Input: part model. Units: mm. Frame: model coordinates. Coordinates: 2 decimals unless noted, no trailing zeros. Loops run counter-clockwise (first coordinate to the right, second up) from the corner with the lowest first, then second, coordinate; pieces in that order, holes last. Notation, with made-up numbers: (-36, -6) - (-22, -6) arc R8 ccw to (-22, 8) - close; hole circle Ø3 at (-6, 43.25). An arc over 180 degrees is marked (long way). Answer as CSV lines item,"result". Start each with the question number.
Autodesk Inventor part; units mm, degrees
ref_plane "YZ Plane" through (0, 0, 0) normal (1, 0, 0) x (0, 1, 0)
ref_plane "XZ Plane" through (0, 0, 0) normal (0, 1, 0) x (-1, 0, 0)
ref_plane "XY Plane" through (0, 0, 0) normal (0, 0, 1) x (1, 0, 0)
sketch "Sketch2" plane through (0, 0, 0) normal (0, 1, 0) x (-1, 0, 0)
  line L0 (0, 0) -> (300, 0)
  line L1 (300, 0) -> (300, -500)
  line L2 (300, -500) -> (0, -500)
  line L3 (0, -500) -> (0, 0)
  line L4 (300, 0) -> (255, 0)
  line L5 (255, 0) -> (255, -45)
  line L6 (255, -45) -> (300, -45)
  line L7 (300, -45) -> (300, 0)
  line L8 (300, -500) -> (255, -500)
  line L9 (255, -500) -> (255, -455)
  line L10 (255, -455) -> (300, -455)
  line L11 (300, -455) -> (300, -500)
  line L12 (0, -500) -> (45, -500)
  line L13 (45, -500) -> (45, -455)
  line L14 (45, -455) -> (0, -455)
  line L15 (0, -455) -> (0, -500)
  line L16 (0, 0) -> (45, 0)
  line L17 (45, 0) -> (45, -45)
  line L18 (45, -45) -> (0, -45)
  line L19 (0, -45) -> (0, 0)
  point P0 (0, -45)
  point P1 (0, -455)
  point P2 (300, -455)
  point P3 (255, 0)
  point P4 (45, 0)
  dimension "d0" = 300
  dimension "d1" = 500
  dimension "d12" = 45
  dimension "d13" = 45
  dimension "d14" = 45
  dimension "d15" = 45
  dimension "d16" = 45
  dimension "d17" = 45
  dimension "d18" = 45
  dimension "d19" = 45
ref_plane "Work Plane1" through (0, 20, 0) normal (0, 1, 0) x (1, 0, 0)
extrude "Extrusion2" add sketch "Sketch2" along normal blind 20 contours L0 L5 L6 L1 L10 L9 L2 L13 L14 L3 L18 L17
properties part number "Shelf"
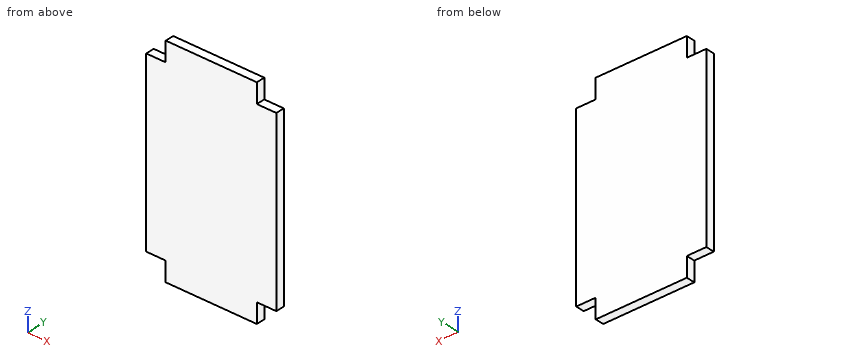
Item 1: Section query A-A, the plane y = 3.5. Output: boundary loops of the cut face in (x, z), and give its area (3 significant figures).
Item 2: Material intervals for probe 1 along X at (y, z) = (11.5, -36.5); probe 2 along Z at (x, y) = (-42, 13.5), sorted ascending.
Item 3: Section query B-B, the plane x = -266.5. Output: boundary loops of the cut face in (y, z).
Item 4: Contact query for flat-ended pins moving along their axis: P1, Ø12, axis at x = -269.5, y = 16, coming from the -Z side; P2, Ø10, axis at y = 12, z = -12, coming from the -X side; P3, Ø10, axis at y = 13.5, z = -26.5, coming from the +X side. Output: stop coordinate, or through.
Response values:
1,outline,"(-300, -455) - (-255, -455) - (-255, -500) - (-45, -500) - (-45, -455) - (0, -455) - (0, -45) - (-45, -45) - (-45, 0) - (-255, 0) - (-255, -45) - (-300, -45) - close"
1,area,"142,000 mm²"
2,probe 1,"x = -255 to -45"
2,probe 2,"z = -455 to -45"
3,outline,"(0, -455) - (20, -455) - (20, -45) - (0, -45) - close"
4,P1,"stops at z = -455"
4,P2,"stops at x = -255"
4,P3,"stops at x = -45"
